Input: part model. Units: mm. Frame: model coordinates. A direction names the side the tool comes from. Give positions to 0.01 mm unless a question says otherwise; leave off trailing zeros. Loops run counter-clockwise (first coordinate to the right, second up) from the corner with the lowest first, then second, coordinate; pieces in that order, holes last. Notation, with made-up numbers: M 30,47.5 L 53,47.5 A5 cw 53,55.5 Z; hole C 75.5,27 d6. An arc over 180 degrees is marked long. One line per item, written item: value. Start each with the question number.
(1) Access query for faces 1 (the flat face through (234.95, 16, 63)), 2 (the flat face through (241.3, 16, 4)), 3 (the flat face through (101.6, 16, -90)). Directions: +Z, -Z, +X, -X, +Y, -Y. A direction counts if a zero-diameter tool reaches every point of the face in a straight line with its end or side. Return the directions, or none.
(2) Section A-A on z = -68.5. Output: boundary loops of the cut face in (x, y).
(3) Section B-B on x = 169.5. Output: boundary loops of the cut face in (y, z) (3 decimals).
(4) Ray query, line 1 along X through (y, z) = (15.75, 56); line 2 along X through (y, z) = (18.75, -55); line 3 along Z through (x, y) = (215.5, 18.75) (3 decimals). Return the intervals inside material, ascending. Write a range as from..to.
(5) Pin query (flat end, axial travel): P1, Ø1.9, axis at y = 17.5, z = 69, coming from the +X side; P2, Ø1.9, axis at y = 15, z = 88.5, coming from the -X side. Return the tip coordinate at first contact, or that it passes through.
```python
from build123d import *

# Parameters (mm, degrees)
SKETCH1_W               = 482.6
SKETCH1_H               = 304.8
BOSS_EXTRUDE1_DEPTH     = 12.7
BOSS_EXTRUDE2_DEPTH     = 6.35
SKETCH3_R               = 1.5875
CUT_EXTRUDE1_DEPTH      = 507.449822292
SKETCH4_W               = 6.35
SKETCH4_H               = 12.7
BOSS_EXTRUDE3_DEPTH     = 292.1
SKETCH5_W               = 12.7
SKETCH5_H               = 19.05
BOSS_EXTRUDE4_DEPTH     = 6.35
CUT_EXTRUDE2_START      = 6.35
CUT_EXTRUDE2_DEPTH      = 25.4
CUT_EXTRUDE3_START      = -488.95
CUT_EXTRUDE3_DEPTH      = 25.4
BOSS_EXTRUDE5_START     = -2.54
BOSS_EXTRUDE5_DEPTH     = 7.62
CUT_EXTRUDE5_DEPTH      = 582.883177708
CUT_EXTRUDE5_DEPTH_BACK = 582.883177708
SKETCH13_W              = 304.8
SKETCH13_H              = 12.7
SKETCH17_W              = 385.398698987
SKETCH17_H              = 324.595378491
CUT_EXTRUDE8_DEPTH      = 291.854955261


with BuildPart() as part:
    # Sketch1 → Boss-Extrude1 (new body)
    with BuildSketch(Plane(origin=(0, 0, 0), x_dir=(1, 0, 0), z_dir=(0, 1, 0))):
        Rectangle(SKETCH1_W, SKETCH1_H)
    extrude(amount=BOSS_EXTRUDE1_DEPTH)

    # Sketch2 → Boss-Extrude2 (add)
    with BuildSketch(Plane(origin=(0, 12.7, 0), x_dir=(1, 0, 0), z_dir=(0, 1, 0))):
        Polygon((-241.3, 152.4), (-234.95, 152.4), (234.95, 152.4), (241.3, 152.4), (241.3, -152.4), (234.95, -152.4), (234.95, 28.575), (-234.95, 28.575), (-234.95, -152.4), (-241.3, -152.4), align=None)
    extrude(amount=BOSS_EXTRUDE2_DEPTH)

    # Sketch3 → Cut-Extrude1 (cut, through all)
    with BuildSketch(Plane.ZY.offset(241.3)):
        with Locations((149.225, 15.875)):
            Circle(SKETCH3_R)
    extrude(amount=-CUT_EXTRUDE1_DEPTH, mode=Mode.SUBTRACT)

    # Sketch4 → Boss-Extrude3 (add)
    with BuildSketch(Plane.XY.offset(152.4)):
        with Locations((-244.475, 6.35)):
            Rectangle(SKETCH4_W, SKETCH4_H)
    boss_extrude3 = extrude(amount=-BOSS_EXTRUDE3_DEPTH)

    # Sketch5 → Boss-Extrude4 (add)
    with BuildSketch(Plane.ZY.offset(241.3)):
        with Locations((-146.05, 9.525)):
            Rectangle(SKETCH5_W, SKETCH5_H)
    boss_extrude4 = extrude(amount=BOSS_EXTRUDE4_DEPTH)

    # Mirror1: Boss-Extrude3, Boss-Extrude4 across plane
    add(boss_extrude3.mirror(Plane(origin=(0, 0, 0), x_dir=(0, 0, 1), z_dir=(1, 0, 0))))
    add(boss_extrude4.mirror(Plane(origin=(0, 0, 0), x_dir=(0, 0, 1), z_dir=(1, 0, 0))))

    # Sketch6 → Cut-Extrude2 (cut)
    with BuildSketch(Plane.ZY.offset(241.3).offset(CUT_EXTRUDE2_START)):
        with BuildLine():
            Line((147.32, 2.54), (128.27, 2.54))
            ThreePointArc((128.27, 2.54), (124.46, 6.35), (128.27, 10.16))
            Line((128.27, 10.16), (147.32, 10.16))
            ThreePointArc((147.32, 10.16), (151.13, 6.35), (147.32, 2.54))
        make_face()
    extrude(amount=-CUT_EXTRUDE2_DEPTH, mode=Mode.SUBTRACT)

    # Sketch6<2> → Cut-Extrude3 (cut)
    with BuildSketch(Plane.ZY.offset(241.3).offset(CUT_EXTRUDE3_START)):
        with BuildLine():
            Line((147.32, 2.54), (128.27, 2.54))
            ThreePointArc((128.27, 2.54), (124.46, 6.35), (128.27, 10.16))
            Line((128.27, 10.16), (147.32, 10.16))
            ThreePointArc((147.32, 10.16), (151.13, 6.35), (147.32, 2.54))
        make_face()
    extrude(amount=CUT_EXTRUDE3_DEPTH, mode=Mode.SUBTRACT)

    # Sketch11 → Boss-Extrude5 (add)
    with BuildSketch(Plane.XZ.offset(BOSS_EXTRUDE5_START)):
        Polygon((-247.65, 124.46), (-222.25, 124.46), (-222.25, 140.97), align=None)
    boss_extrude5 = extrude(amount=-BOSS_EXTRUDE5_DEPTH)

    # Mirror2: Boss-Extrude5 across plane
    add(boss_extrude5.mirror(Plane(origin=(0, 0, 0), x_dir=(0, 0, 1), z_dir=(1, 0, 0))))

    # Sketch13 → Cut-Extrude5 (cut, two sides: drawn at the far end of the back side and taken through both)
    with BuildSketch(Plane(origin=(247.65, 19.05, -152.4), x_dir=(0, 0, 1), z_dir=(-1, 0, 0)).offset(-CUT_EXTRUDE5_DEPTH_BACK)):
        with Locations((152.4, -12.7)):
            Rectangle(SKETCH13_W, SKETCH13_H)
    extrude(amount=CUT_EXTRUDE5_DEPTH + CUT_EXTRUDE5_DEPTH_BACK, mode=Mode.SUBTRACT)

    # Sketch17 → Cut-Extrude8 (cut, through all)
    with BuildSketch(Plane(origin=(0, 19.05, 0), x_dir=(1, 0, 0), z_dir=(0, 1, 0))):
        with Locations((-91.099349494, -9.897689246)):
            Rectangle(SKETCH17_W, SKETCH17_H)
    extrude(amount=-CUT_EXTRUDE8_DEPTH, mode=Mode.SUBTRACT)


solid = part.part
```
Output values:
1. face 1: +Z, -X, +Y, -Y
1. face 2: +Z, +X, +Y, -Y
1. face 3: +Z, -Z, -X, +Y, -Y
2. outline: M 101.6,12.7 L 241.3,12.7 L 241.3,19.05 L 101.6,19.05 Z
3. outline: M 12.7,-152.4 L 19.05,-152.4 L 19.05,-28.575 L 12.7,-28.575 Z
4. line 1: x = 234.95..241.3
4. line 2: x = 101.6..241.3
4. line 3: z = -152.4..-28.575
5. P1: stops at x = 241.3
5. P2: stops at x = 234.95
